Can you work these out from the model? Positions are in its coordinate system, mm. A direction names the side the tool comes from. Round coordinates to 2 decimals unless told otherwise and drop trailing zeros. Order: outer loops, then holes, each group sorted by start corner. A loop starts at its lowest first (then second) coordinate and runs counter-clockwise, first axis right, second up. Notation, with made-up numbers: M 12,37.5 L 43,37.5 A14 cw 43,57.5 Z; hole C -25,61 d6. An arc over 180 degrees is marked long. Answer as a JSON object with one key per item and string values. Group by question number.
from build123d import *

# Parameters (mm, degrees)
F1_DEPTH       = 134
F3_D           = 4
F3_CBORE_D     = 9.75
F3_CBORE_DEPTH = 5
F4_R           = 7
F5_DEPTH       = 4
F6_R           = 7
F7_DEPTH       = 7
F7_TAPER       = 40


with BuildPart() as f1:
    # F0 (on Front) → F1 (new body)
    with BuildSketch(Plane.XZ):
        Polygon((23.5, 0), (0, 0), (0, -1), (10.25, -8.8510638298), (13.25, -8.8510638298), (23.5, -1), align=None)
    extrude(amount=F1_DEPTH)

    # F3 (through all)
    with Locations(Plane.XY):
        with Locations((11.75, -15), (11.75, -67), (11.75, -119)):
            CounterBoreHole(F3_D / 2, F3_CBORE_D / 2, F3_CBORE_DEPTH)

    # F4 (on face) → F5 (join)
    with BuildSketch(Plane.XY):
        with Locations((11.75, -40)):
            Circle(F4_R)
        with Locations((11.75, -94)):
            Circle(F4_R)
    extrude(amount=F5_DEPTH)

    # F6 (on face) → F7 (join)
    with BuildSketch(Plane.XY.offset(4)):
        with Locations((11.75, -40)):
            Circle(F6_R)
        with Locations((11.75, -94)):
            Circle(F6_R)
    extrude(amount=F7_DEPTH, taper=F7_TAPER)


solid = f1.part
Item 1: On a 3-axis mill with a long thin cutter (end or side, diameter ignored), from which of +Z, -Z, +X, -X, +Y, -Y can I reach the whole of each face in a straight line? I mean faces 1 (the face through (11.115, -62.166, -2.465)), 2 (the face through (5.05, -66.06, -4.87)). Say none if no direction works.
Item 2: I'm going to push flat-ended pins straight in: pin 1 Ø1 at (x, y) = (17, -92) entering from -Z; pin 2 Ø8 at (x, y) = (11.75, -15) entering from +Z; pin 3 Ø7 at (x, y) = (8.5, -59.5) entering from +Z; pin 4 Ø3.5 at (x, y) = (11.75, -119) entering from -Z. Where does each tip first touch, or does it pass through?
Item 3: Suppose I cut it at B-B, the plane y = -40. Write out the boundary of the cut face in (x, z).
Item 4: If we mould it in two halves opening along Y, with no side actions, what happens to faces 3 (the face through (12, -93, -8.851)), 4 (the face through (7.881, -17.966, -2.465)), 5 (the face through (12, -134, -3)), 6 (the face through (10.84, -87.06, 1.97))? For each: +Y half, -Y half, draft (parallel to the pull), parting line (faces both ways), or undercut.
Item 5: Suppose I cut it at C-C, the plane z = 7. Write out the boundary of the cut face in (x, y), and give its area (3 significant figures).
Item 6: Suppose I cut it at A-A, the plane y = -15. Write out the boundary of the cut face in (x, z) (3 decimals).
Item 7: I need wall thicknesses on line 1 (Y direction, x = 11.75, z = -5.85); line 2 (Y direction, x = 11.75, z = -1.4) (3 decimals); line 3 (X direction, y = -67, z = -7.6). Which ranges of each line are inside material? Lowest first, please.
Computed:
{
 "1": {"face 1": "+Z", "face 2": "-Z, -X, +Y, -Y"},
 "2": {"pin 1": "stops at z = -6.36", "pin 2": "stops at z = -5", "pin 3": "stops at z = 0", "pin 4": "passes through"},
 "3": {"outline": "M 0,-1 L 10.25,-8.85 L 13.25,-8.85 L 23.5,-1 L 23.5,0 L 18.75,0 L 18.75,4 L 12.88,11 L 10.62,11 L 4.75,4 L 4.75,0 L 0,0 Z"},
 "4": {"face 3": "draft", "face 4": "undercut", "face 5": "-Y half", "face 6": "undercut"},
 "5": {"outline": "C 11.75,-94 d8.97; C 11.75,-40 d8.97", "area": "126 mm^2"},
 "6": {"outline": "M 0,-1 L 9.75,-8.468 L 9.75,-5 L 6.875,-5 L 6.875,0 L 0,0 Z; M 13.75,-8.468 L 23.5,-1 L 23.5,0 L 16.625,0 L 16.625,-5 L 13.75,-5 Z"},
 "7": {"line 1": "y = -134 to -121, -117 to -69, -65 to -17, -13 to 0", "line 2": "y = -134 to -123.875, -114.125 to -71.875, -62.125 to -19.875, -10.125 to 0", "line 3": "x = 8.62 to 9.75, 13.75 to 14.88"}
}
